Here's how the part is built. I have some questions about the finished solid (model axes, mm). Face numbers are marked on the shaded views. A direction names the side the tool comes from. Coordinates: 2 decimals unless noted, no trailing zeros. Order: outer loops, then holes, each group sorted by start corner. A loop starts at its lowest first (then second) coordinate and runs counter-clockwise, first axis right, second up.
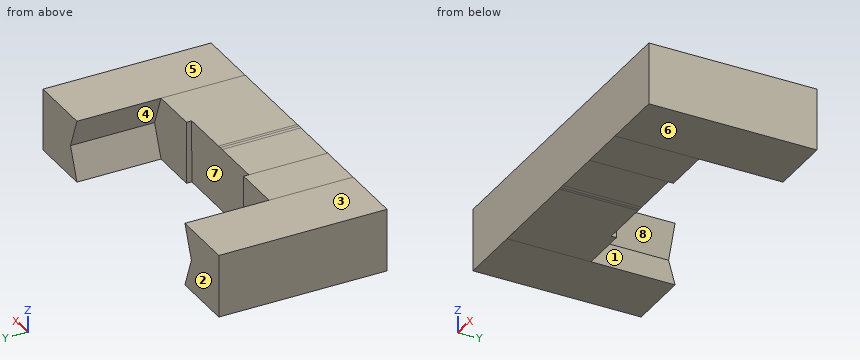
```python
from build123d import *

# Parameters (mm, degrees)
F1_DEPTH = 8
F2_DEPTH = 4
F3_DEPTH = 4.25


# Not quite as in the source:
# - a feature of the source that left no trace in its solid (it failed there, or was rolled back) is left out


with BuildPart() as f1:
    # F0 (on Front) → F1 (new body)
    with BuildSketch(Plane.XZ):
        with BuildLine():
            Line((2.5197209473, -1.4865167008), (2.5252201747, 1.4865065289))
            Line((2.5252201747, 1.4865065289), (0.1652307775, 1.4908718222))
            ThreePointArc((0.1652307775, 1.4908718222), (1.1175522731, 1.0005383135), (1.5, 0))
            ThreePointArc((1.5, 0), (1.1175522731, -1.0005383135), (0.1652307775, -1.4908718222))
            Line((0.1652307775, -1.4908718222), (2.5197209473, -1.4865167008))
        make_face()
        Polygon((-5.3444080986, 0), (-4.7696960071, 1.5), (-7.7696960071, 1.5), (-7.7696960071, -1.5), (-4.7696960071, -1.5), align=None)
        Polygon((7.7752124765, 1.4823446982), (4.7752124765, 1.4823446982), (5.3444080986, 0), (4.7752124765, -1.4823446982), (7.7752124765, -1.4823446982), align=None)
        with BuildLine():
            ThreePointArc((-4.7696960071, -1.5), (-5, 0), (-4.7696960071, 1.5))
            Line((-4.7696960071, 1.5), (-5.3444080986, 0))
            Line((-5.3444080986, 0), (-4.7696960071, -1.5))
        make_face()
        with BuildLine():
            Line((5.3444080986, 0), (4.7752124765, 1.4823446982))
            ThreePointArc((4.7752124765, 1.4823446982), (4.94348371, 0.7496457888), (5, 0))
            ThreePointArc((5, 0), (4.94348371, -0.7496457888), (4.7752124765, -1.4823446982))
            Line((4.7752124765, -1.4823446982), (5.3444080986, 0))
        make_face()
        with BuildLine():
            Line((-2.5252374544, 1.4958484051), (-4.7696960071, 1.5))
            ThreePointArc((-4.7696960071, 1.5), (-5, 0), (-4.7696960071, -1.5))
            Line((-4.7696960071, -1.5), (-2.5197037053, -1.4958381693))
            Line((-2.5197037053, -1.4958381693), (-2.5252374544, 1.4958484051))
        make_face()
        with BuildLine():
            ThreePointArc((5, 0), (4.94348371, 0.7496457888), (4.7752124765, 1.4823446982))
            Line((4.7752124765, 1.4823446982), (2.5252201747, 1.4865065289))
            Line((2.5252201747, 1.4865065289), (2.5197209473, -1.4865167008))
            Line((2.5197209473, -1.4865167008), (4.7752124765, -1.4823446982))
            ThreePointArc((4.7752124765, -1.4823446982), (4.94348371, -0.7496457888), (5, 0))
        make_face()
        with BuildLine():
            Line((0, 1.491177451), (-0.1597143081, 1.491472876))
            ThreePointArc((-0.1597143081, 1.491472876), (-1.5, 0), (-0.1597143081, -1.491472876))
            Line((-0.1597143081, -1.491472876), (0, -1.491177451))
            Line((0, -1.491177451), (0, 1.491177451))
        make_face()
        with BuildLine():
            Line((-0.1597143081, 1.491472876), (-2.5252374544, 1.4958484051))
            Line((-2.5252374544, 1.4958484051), (-2.5197037053, -1.4958381693))
            Line((-2.5197037053, -1.4958381693), (-0.1597143081, -1.491472876))
            ThreePointArc((-0.1597143081, -1.491472876), (-1.5, 0), (-0.1597143081, 1.491472876))
        make_face()
        with BuildLine():
            ThreePointArc((1.5, 0), (1.1175522731, 1.0005383135), (0.1652307775, 1.4908718222))
            Line((0.1652307775, 1.4908718222), (0, 1.491177451))
            Line((0, 1.491177451), (0, -1.491177451))
            Line((0, -1.491177451), (0.1652307775, -1.4908718222))
            ThreePointArc((0.1652307775, -1.4908718222), (1.1175522731, -1.0005383135), (1.5, 0))
        make_face()
        with BuildLine():
            Line((0, 1.491177451), (0.1652307775, 1.4908718222))
            ThreePointArc((0.1652307775, 1.4908718222), (0.0827413643, 1.497716217), (0, 1.5))
            Line((0, 1.5), (0, 1.491177451))
        make_face()
        with BuildLine():
            ThreePointArc((0, 1.5), (-0.0799708885, 1.497866702), (-0.1597143081, 1.491472876))
            Line((-0.1597143081, 1.491472876), (0, 1.491177451))
            Line((0, 1.491177451), (0, 1.5))
        make_face()
        with BuildLine():
            Line((0, -1.491177451), (-0.1597143081, -1.491472876))
            ThreePointArc((-0.1597143081, -1.491472876), (-0.0799708885, -1.497866702), (0, -1.5))
            Line((0, -1.5), (0, -1.491177451))
        make_face()
        with BuildLine():
            ThreePointArc((0, -1.5), (0.0827413643, -1.497716217), (0.1652307775, -1.4908718222))
            Line((0.1652307775, -1.4908718222), (0, -1.491177451))
            Line((0, -1.491177451), (0, -1.5))
        make_face()
    extrude(amount=F1_DEPTH)

    # F0 (on Front) → F2 (cut)
    with BuildSketch(Plane.XZ):
        with BuildLine():
            Line((5.3444080986, 0), (4.7752124765, 1.4823446982))
            ThreePointArc((4.7752124765, 1.4823446982), (4.94348371, 0.7496457888), (5, 0))
            ThreePointArc((5, 0), (4.94348371, -0.7496457888), (4.7752124765, -1.4823446982))
            Line((4.7752124765, -1.4823446982), (5.3444080986, 0))
        make_face()
        with BuildLine():
            ThreePointArc((5, 0), (4.94348371, 0.7496457888), (4.7752124765, 1.4823446982))
            Line((4.7752124765, 1.4823446982), (2.5252201747, 1.4865065289))
            Line((2.5252201747, 1.4865065289), (2.5197209473, -1.4865167008))
            Line((2.5197209473, -1.4865167008), (4.7752124765, -1.4823446982))
            ThreePointArc((4.7752124765, -1.4823446982), (4.94348371, -0.7496457888), (5, 0))
        make_face()
        with BuildLine():
            Line((2.5197209473, -1.4865167008), (2.5252201747, 1.4865065289))
            Line((2.5252201747, 1.4865065289), (0.1652307775, 1.4908718222))
            ThreePointArc((0.1652307775, 1.4908718222), (1.1175522731, 1.0005383135), (1.5, 0))
            ThreePointArc((1.5, 0), (1.1175522731, -1.0005383135), (0.1652307775, -1.4908718222))
            Line((0.1652307775, -1.4908718222), (2.5197209473, -1.4865167008))
        make_face()
        with BuildLine():
            ThreePointArc((1.5, 0), (1.1175522731, 1.0005383135), (0.1652307775, 1.4908718222))
            Line((0.1652307775, 1.4908718222), (0, 1.491177451))
            Line((0, 1.491177451), (0, -1.491177451))
            Line((0, -1.491177451), (0.1652307775, -1.4908718222))
            ThreePointArc((0.1652307775, -1.4908718222), (1.1175522731, -1.0005383135), (1.5, 0))
        make_face()
        with BuildLine():
            Line((0, 1.491177451), (-0.1597143081, 1.491472876))
            ThreePointArc((-0.1597143081, 1.491472876), (-1.5, 0), (-0.1597143081, -1.491472876))
            Line((-0.1597143081, -1.491472876), (0, -1.491177451))
            Line((0, -1.491177451), (0, 1.491177451))
        make_face()
        with BuildLine():
            Line((-0.1597143081, 1.491472876), (-2.5252374544, 1.4958484051))
            Line((-2.5252374544, 1.4958484051), (-2.5197037053, -1.4958381693))
            Line((-2.5197037053, -1.4958381693), (-0.1597143081, -1.491472876))
            ThreePointArc((-0.1597143081, -1.491472876), (-1.5, 0), (-0.1597143081, 1.491472876))
        make_face()
        with BuildLine():
            Line((-2.5252374544, 1.4958484051), (-4.7696960071, 1.5))
            ThreePointArc((-4.7696960071, 1.5), (-5, 0), (-4.7696960071, -1.5))
            Line((-4.7696960071, -1.5), (-2.5197037053, -1.4958381693))
            Line((-2.5197037053, -1.4958381693), (-2.5252374544, 1.4958484051))
        make_face()
        with BuildLine():
            ThreePointArc((-4.7696960071, -1.5), (-5, 0), (-4.7696960071, 1.5))
            Line((-4.7696960071, 1.5), (-5.3444080986, 0))
            Line((-5.3444080986, 0), (-4.7696960071, -1.5))
        make_face()
    extrude(amount=F2_DEPTH, mode=Mode.SUBTRACT)

    # F0 (on Front) → F3 (cut)
    with BuildSketch(Plane.XZ):
        with BuildLine():
            Line((2.5197209473, -1.4865167008), (2.5252201747, 1.4865065289))
            Line((2.5252201747, 1.4865065289), (0.1652307775, 1.4908718222))
            ThreePointArc((0.1652307775, 1.4908718222), (1.1175522731, 1.0005383135), (1.5, 0))
            ThreePointArc((1.5, 0), (1.1175522731, -1.0005383135), (0.1652307775, -1.4908718222))
            Line((0.1652307775, -1.4908718222), (2.5197209473, -1.4865167008))
        make_face()
        with BuildLine():
            ThreePointArc((1.5, 0), (1.1175522731, 1.0005383135), (0.1652307775, 1.4908718222))
            Line((0.1652307775, 1.4908718222), (0, 1.491177451))
            Line((0, 1.491177451), (0, -1.491177451))
            Line((0, -1.491177451), (0.1652307775, -1.4908718222))
            ThreePointArc((0.1652307775, -1.4908718222), (1.1175522731, -1.0005383135), (1.5, 0))
        make_face()
        with BuildLine():
            Line((-0.1597143081, 1.491472876), (-2.5252374544, 1.4958484051))
            Line((-2.5252374544, 1.4958484051), (-2.5197037053, -1.4958381693))
            Line((-2.5197037053, -1.4958381693), (-0.1597143081, -1.491472876))
            ThreePointArc((-0.1597143081, -1.491472876), (-1.5, 0), (-0.1597143081, 1.491472876))
        make_face()
        with BuildLine():
            Line((0, 1.491177451), (-0.1597143081, 1.491472876))
            ThreePointArc((-0.1597143081, 1.491472876), (-1.5, 0), (-0.1597143081, -1.491472876))
            Line((-0.1597143081, -1.491472876), (0, -1.491177451))
            Line((0, -1.491177451), (0, 1.491177451))
        make_face()
        with BuildLine():
            ThreePointArc((0, 1.5), (-0.0799708885, 1.497866702), (-0.1597143081, 1.491472876))
            Line((-0.1597143081, 1.491472876), (0, 1.491177451))
            Line((0, 1.491177451), (0, 1.5))
        make_face()
        with BuildLine():
            Line((0, 1.491177451), (0.1652307775, 1.4908718222))
            ThreePointArc((0.1652307775, 1.4908718222), (0.0827413643, 1.497716217), (0, 1.5))
            Line((0, 1.5), (0, 1.491177451))
        make_face()
        with BuildLine():
            ThreePointArc((0, -1.5), (0.0827413643, -1.497716217), (0.1652307775, -1.4908718222))
            Line((0.1652307775, -1.4908718222), (0, -1.491177451))
            Line((0, -1.491177451), (0, -1.5))
        make_face()
        with BuildLine():
            Line((0, -1.491177451), (-0.1597143081, -1.491472876))
            ThreePointArc((-0.1597143081, -1.491472876), (-0.0799708885, -1.497866702), (0, -1.5))
            Line((0, -1.5), (0, -1.491177451))
        make_face()
    extrude(amount=F3_DEPTH, mode=Mode.SUBTRACT)


solid = f1.part
```
Q1. We'd pull the mould along Z, two halves only. Please class the marked faces 1, 2, 3 and 4: pulls with the +Z half, pulls with the -Z half, needs draft (parallel to the pull), parting line crosses it, or undercut.
Q2. If we section it at D-D on x = 0.75: Write out the boundary of the cut face in (y, z), then the cut area to 3 significant figures.
Q3. Will these pins go through, and if not, where does the flat tip stop? pin 1 (2.5 mm diameter, centred on x = 7, y = -3, fed in from -Z); pin 2 (0.9 mm diameter, centred on x = 0, z = -0.5, fed in from +Y); pin 3 (1.4 mm diameter, centred on x = 4.5, z = 0, fed in from +Y).
Q4. I need wall thicknesses on L1, parallel to Y at x = -1.25, z = 0.8; L2, parallel to Z at x = 6.5, y = -1; L3, parallel to X at y = -1.5, z = -0.25. Which ranges of each line are inside material? Lowest first, please.
Q5. If we section it at B-B on z = 0.3: Write out the boundary of the cut face in (x, y), then the cut area to 3 significant figures.
Q6. If we section it at A-A on y = -1: Write out the boundary of the cut face in (x, z).
Q7. If we section it at C-C on x = -3.25: Write out the boundary of the cut face in (y, z).
Q8. For the marked faces 5, 6, 7 and 8, which set-ups out of +Z, -Z, +X, -X, +Y, -Y let a thin tool reach every point of the face, with its end or its side?
Reply:
1. face 1: undercut
1. face 2: needs draft
1. face 3: pulls with the +Z half
1. face 4: undercut
2. outline: (-8, -1.49) - (-4.25, -1.49) - (-4.25, 1.49) - (-8, 1.49) - close
2. area: 11.2 mm2
3. pin 1: stops at z = -1.48
3. pin 2: stops at y = -4.25
3. pin 3: stops at y = -4
4. L1: y = -8 to -4.25
4. L2: z = -1.48 to 1.48
4. L3: x = -7.77 to -5.25, 5.25 to 7.78
5. outline: (-7.77, -8) - (7.78, -8) - (7.78, 0) - (5.23, 0) - (5.23, -4) - (2.52, -4) - (2.52, -4.25) - (-2.52, -4.25) - (-2.52, -4) - (-5.23, -4) - (-5.23, 0) - (-7.77, 0) - close
5. area: 81.3 mm2
6. outline: (-7.77, -1.5) - (-4.77, -1.5) - (-5.34, 0) - (-4.77, 1.5) - (-7.77, 1.5) - close; (4.78, -1.48) - (7.78, -1.48) - (7.78, 1.48) - (4.78, 1.48) - (5.34, 0) - close
7. outline: (-8, -1.5) - (-4, -1.5) - (-4, 1.5) - (-8, 1.5) - close
8. face 5: +Z, +X, +Y, -Y
8. face 6: -Z, +X, +Y, -Y
8. face 7: +Z, -Z, +Y
8. face 8: +Y
